Work out the finished part from the listing and answer in its coordinate system (mm). Give positions to 0.01 mm unless a question says otherwise; leave off trailing zeros. Write each loop counter-clockwise with the first axis right and the second up, starting at its lowest first coordinate (ties: lowest second). Pieces come first, ordered by that corner, then holes. Notation, with made-up numbers: (19.25, -36) - (57.25, -36) arc R19 ccw to (57.25, -3) - close; hole circle Ø3 at (-32.5, 9). An arc over 180 degrees is marked (long way). Write item = value, one per line.
from build123d import *

# Parameters (mm, degrees)
F0_W     = 27.3773
F0_H     = 35.429452
F1_DEPTH = 6.18124
F2_R     = 5
F3_R     = 1.216032
F4_DEPTH = 25


with BuildPart() as f1:
    # F0 (on Top) → F1 (new body)
    with BuildSketch(Plane.XY):
        with Locations((-34.624234, 32.047549)):
            Rectangle(F0_W, F0_H)
    extrude(amount=F1_DEPTH)

    # F2
    f2_edges = [f1.edges().sort_by_distance(p)[0] for p in [
        (-20.935584, 49.762275, 3.09062),
        (-48.312884, 49.762275, 3.09062),
    ]]
    fillet(f2_edges, radius=F2_R)

    # F3 (on Top) → F4 (cut)
    with BuildSketch(Plane.XY):
        with Locations((-35.054151, 43.442421)):
            Circle(F3_R)
    extrude(amount=F4_DEPTH, mode=Mode.SUBTRACT)


solid = f1.part
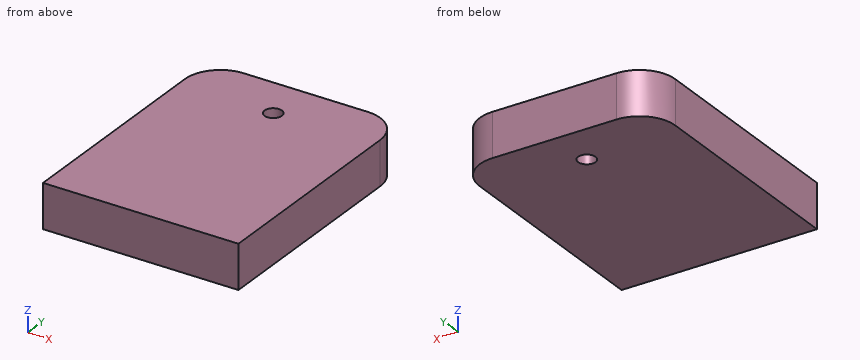
1. Find section A-A, the plane z = 4.5. Give the vertices of the cut face in (x, y), then the cut area to 3 significant figures.
Solution:
outline = (-48.31, 14.33) - (-20.94, 14.33) - (-20.94, 44.76) arc R5 ccw to (-25.94, 49.76) - (-43.31, 49.76) arc R5 ccw to (-48.31, 44.76) - close; hole circle Ø2.43 at (-35.05, 43.44)
area = 955 mm^2
2. Find section C-C, the plane y = 47.5. Give the vertices of the cut face in (x, z), then the cut area to 3 significant figures.
Solution:
outline = (-47.5, 0) - (-21.75, 0) - (-21.75, 6.18) - (-47.5, 6.18) - close
area = 159 mm^2
3. Find section B-B, the plane x = -23.25. Give the vertices of the cut face in (y, z).
Solution:
outline = (14.33, 0) - (48.98, 0) - (48.98, 6.18) - (14.33, 6.18) - close
4. Straight lines are drawn through the part: line 1 (X direction, y = 46, z = 5.5); line 2 (X direction, y = 43, z = 1); line 3 (Y direction, x = -34, z = 0.75). For each, find the intervals that lie inside material, in ascending order.
Solution:
line_1 = -48.16 to -21.09
line_2 = -48.31 to -36.19, -33.92 to -20.94
line_3 = 14.33 to 42.84, 44.05 to 49.76
